Check sheet for the modelled part. Datum: model origin and axes. Units: mm. A direction names the side the tool comes from. Round coordinates to 2 decimals unless told otherwise and drop trailing zeros. Order: outer loops, then holes, each group sorted by start corner. A loop starts at its lowest first (then second) coordinate and runs counter-clockwise, first axis right, second up.
from build123d import *

# Parameters (mm, degrees)
SKETCH_1_W                         = 2.79
SKETCH_1_H                         = 5
EXTRUDE_1_DEPTH                    = 8.4
SKETCH_2_W                         = 1
SKETCH_2_H                         = 1
CUT_EXTRUDE_1_DEPTH                = 8
CHAMFER_1_SIZE                     = 0.2
SKETCH_3_W                         = 0.64
SKETCH_3_H                         = 0.64
EXTRUDE_2_DEPTH                    = 2.29
CHAMFER_2_SIZE                     = 0.2
PATTERN_LINEAR_1_COUNT             = 2
PATTERN_LINEAR_1_PITCH             = 2.54
CHAMFER_1_OF_PATTERN_LINEAR_1_SIZE = 0.2
CHAMFER_2_OF_PATTERN_LINEAR_1_SIZE = 0.2


with BuildPart() as part:
    # Эскиз1 → Бобышка-Вытянуть1 (new body)
    with BuildSketch(Plane(origin=(0, 0, 0), x_dir=(1, 0, 0), z_dir=(0, 1, 0))):
        Rectangle(SKETCH_1_W, SKETCH_1_H)
    extrude_1 = extrude(amount=EXTRUDE_1_DEPTH)

    # Эскиз2 → Вырез-Вытянуть1 (cut)
    with BuildSketch(Plane(origin=(0, 8.4, 0), x_dir=(1, 0, 0), z_dir=(0, 1, 0))):
        with Locations((0, 1.27)):
            Rectangle(SKETCH_2_W, SKETCH_2_H)
        with Locations((0, -1.27)):
            Rectangle(SKETCH_2_W, SKETCH_2_H)
    cut_extrude_1 = extrude(amount=-CUT_EXTRUDE_1_DEPTH, mode=Mode.SUBTRACT)

    # Фаска1
    chamfer_1_edges = [part.edges().sort_by_distance(p)[0] for p in [
        (0.5, 8.4, -1.27),
        (0, 8.4, -1.77),
        (-0.5, 8.4, -1.27),
        (0, 8.4, -0.77),
        (0, 8.4, 1.77),
        (0.5, 8.4, 1.27),
        (0, 8.4, 0.77),
        (-0.5, 8.4, 1.27),
    ]]
    chamfer(chamfer_1_edges, length=CHAMFER_1_SIZE)

    # Эскиз3 → Бобышка-Вытянуть2 (add)
    with BuildSketch(Plane(origin=(0, 0, 0), x_dir=(-1, 0, 0), z_dir=(0, -1, 0))):
        with Locations((0, 1.27)):
            Rectangle(SKETCH_3_W, SKETCH_3_H)
        with Locations((0, -1.27)):
            Rectangle(SKETCH_3_W, SKETCH_3_H)
    extrude_2 = extrude(amount=EXTRUDE_2_DEPTH)

    # Фаска2
    chamfer_2_edges = [part.edges().sort_by_distance(p)[0] for p in [
        (0.32, -2.29, -1.27),
        (0, -2.29, -0.95),
        (-0.32, -2.29, -1.27),
        (0, -2.29, -1.59),
        (-0.32, -2.29, 1.27),
        (0, -2.29, 0.95),
        (0.32, -2.29, 1.27),
        (0, -2.29, 1.59),
    ]]
    chamfer(chamfer_2_edges, length=CHAMFER_2_SIZE)

    # Линейный массив1: Бобышка-Вытянуть1, Вырез-Вытянуть1, Бобышка-Вытянуть2 ×2
    with Locations(*[(i * PATTERN_LINEAR_1_PITCH, 0, 0) for i in range(1, PATTERN_LINEAR_1_COUNT)]):
        add(extrude_1)
        add(cut_extrude_1, mode=Mode.SUBTRACT)
        add(extrude_2)

    # Фаска1 of Линейный массив1
    chamfer_1_of_pattern_linear_1_edges = [part.edges().sort_by_distance(p)[0] for p in [
        (3.04, 8.4, -1.27),
        (2.54, 8.4, -1.77),
        (2.04, 8.4, -1.27),
        (2.54, 8.4, -0.77),
        (2.54, 8.4, 1.77),
        (3.04, 8.4, 1.27),
        (2.54, 8.4, 0.77),
        (2.04, 8.4, 1.27),
    ]]
    chamfer(chamfer_1_of_pattern_linear_1_edges, length=CHAMFER_1_OF_PATTERN_LINEAR_1_SIZE)

    # Фаска2 of Линейный массив1
    chamfer_2_of_pattern_linear_1_edges = [part.edges().sort_by_distance(p)[0] for p in [
        (2.86, -2.29, -1.27),
        (2.54, -2.29, -0.95),
        (2.22, -2.29, -1.27),
        (2.54, -2.29, -1.59),
        (2.22, -2.29, 1.27),
        (2.54, -2.29, 0.95),
        (2.86, -2.29, 1.27),
        (2.54, -2.29, 1.59),
    ]]
    chamfer(chamfer_2_of_pattern_linear_1_edges, length=CHAMFER_2_OF_PATTERN_LINEAR_1_SIZE)


solid = part.part
1) Sectioned sample at D-D on z = 2.15. Record the cut outline in (x, y) (3 decimals), and give its area (3 significant figures).
2) Set-up check for faces 4 (the face through (1, 8.4, 0)), 5 (the face through (0, 0.4, -1)): record each of +Z, -Z, +X, -X, +Y, -Y from which the full face is reachable in a straight line by a thin tool's end or side.
3) Sectioned sample at A-A on y = -0.25. Record the cut outline in (x, z), and give its area (3 significant figures).
4) Draft check along X on faces 1 (the face through (1, 4, 2.5)), 2 (the face through (0.5, 4, 1)), 3 (the face through (3.935, 4, 0)). Enter one of: pulls with the +X half, pulls with the -X half, needs draft (parallel to the pull), parting line crosses it, or undercut.
5) Sectioned sample at B-B on y = 5.75. Record the cut outline in (x, z) (3 decimals), and give its area (4 significant figures).
6) Sectioned sample at C-C on x = 0.9. Record the cut outline in (y, z), and give its area (3 significant figures).
7) Scan lines: line 1 (X direction, y = 5.75, z = -1.5) (3 decimals); line 2 (Z direction, x = 2.55, y = -0.5); line 3 (Y direction, x = 2.65, z = -2.25). Record each from-to range of solid material in increasing order.
8) Gauge pin test, flat ends, axial feed: pin 1 (0.7 mm diameter, centred on x = 2.5, y = -1.5, fed in from +Z); pin 2 (0.5 mm diameter, centred on y = -1, z = -1.5, fed in from -X); pin 3 (0.5 mm diameter, centred on x = 0, y = -1.5, fed in from -Z); pin 4 (1.5 mm diameter, centred on x = 2, y = -0.5, fed in from +Z). Record the tip position at first contact, or that the pin passes through.
Values found:
1. outline: (-1.395, 0) - (3.935, 0) - (3.935, 8.4) - (-1.395, 8.4) - close
1. area: 44.8 mm2
2. face 4: +Z, -Z, +X, -X, +Y
2. face 5: +Y
3. outline: (-0.32, -1.59) - (0.32, -1.59) - (0.32, -0.95) - (-0.32, -0.95) - close; (-0.32, 0.95) - (0.32, 0.95) - (0.32, 1.59) - (-0.32, 1.59) - close; (2.22, -1.59) - (2.86, -1.59) - (2.86, -0.95) - (2.22, -0.95) - close; (2.22, 0.95) - (2.86, 0.95) - (2.86, 1.59) - (2.22, 1.59) - close
3. area: 1.64 mm2
4. face 1: needs draft
4. face 2: undercut
4. face 3: pulls with the +X half
5. outline: (-1.395, -2.5) - (3.935, -2.5) - (3.935, 2.5) - (-1.395, 2.5) - close; hole (-0.5, -1.77) - (0.5, -1.77) - (0.5, -0.77) - (-0.5, -0.77) - close; hole (-0.5, 0.77) - (0.5, 0.77) - (0.5, 1.77) - (-0.5, 1.77) - close; hole (2.04, -1.77) - (3.04, -1.77) - (3.04, -0.77) - (2.04, -0.77) - close; hole (2.04, 0.77) - (3.04, 0.77) - (3.04, 1.77) - (2.04, 1.77) - close
5. area: 22.65 mm2
6. outline: (0, -2.5) - (8.4, -2.5) - (8.4, 2.5) - (0, 2.5) - close
6. area: 42.0 mm2
7. line 1: x = -1.395 to -0.5, 0.5 to 2.04, 3.04 to 3.935
7. line 2: z = -1.59 to -0.95, 0.95 to 1.59
7. line 3: y = 0 to 8.4
8. pin 1: stops at z = 1.59
8. pin 2: stops at x = -0.32
8. pin 3: stops at z = -1.59
8. pin 4: stops at z = 2.5
